Source: CAD feature listing. Evaluate the final solid. Frame: model axes, mm. A direction names the side the tool comes from. Give positions to 0.01 mm unless a question says otherwise; leave off trailing zeros. Loops run counter-clockwise (first coordinate to the right, second up) from the corner with the lowest first, then second, coordinate; pieces in that order, holes last. Notation, with made-up numbers: M 73.25,85.5 L 93.25,85.5 A16 cw 93.25,112.5 Z; hole C -6,22.5 d8. An arc over 180 degrees is marked long. Put each result on its own line as item: value.
from build123d import *

# Parameters (mm, degrees)
SKIZZE2_W                       = 113.5
SKIZZE2_H                       = 71
AUFSATZ_LINEAR_AUSTRAGEN1_DEPTH = 1.3
AUFSATZ_LINEAR_START            = -0.9
SKIZZE3_W                       = 120.5
SKIZZE3_H                       = 77.2
AUFSATZ_LINEAR_AUSTRAGEN2_DEPTH = 0.4
SKIZZE4_W                       = 107.4
SKIZZE4_H                       = 65
SCHNITT_LINEAR_AUSTRAGEN1_DEPTH = 103.975737434
VERRUNDUNG1_R                   = 1.5
VERRUNDUNG2_R                   = 3.3
VERRUNDUNG3_R                   = 3
SKIZZE5_R                       = 2.9
SCHNITT_LINEAR_AUSTRAGEN2_DEPTH = 103.975737434


with BuildPart() as part:
    # Skizze2 → Aufsatz-Linear austragen1 (new body)
    with BuildSketch(Plane.XY.offset(19.9)):
        with Locations((0, 46.4)):
            Rectangle(SKIZZE2_W, SKIZZE2_H)
    extrude(amount=-AUFSATZ_LINEAR_AUSTRAGEN1_DEPTH)

    # Skizze3 → Aufsatz-Linear austragen2 (add)
    with BuildSketch(Plane.XY.offset(19.9).offset(AUFSATZ_LINEAR_START)):
        with Locations((0, 44.9)):
            Rectangle(SKIZZE3_W, SKIZZE3_H)
    extrude(amount=-AUFSATZ_LINEAR_AUSTRAGEN2_DEPTH)

    # Skizze4 → Schnitt-Linear austragen1 (cut, through all)
    with BuildSketch(Plane.XY.offset(19.9)):
        with Locations((0, 46.4)):
            Rectangle(SKIZZE4_W, SKIZZE4_H)
    extrude(amount=-SCHNITT_LINEAR_AUSTRAGEN1_DEPTH, mode=Mode.SUBTRACT)

    # Verrundung1
    verrundung1_edges = [part.edges().sort_by_distance(p)[0] for p in [
        (56.75, 81.9, 19.45),
        (-56.75, 81.9, 19.45),
    ]]
    fillet(verrundung1_edges, radius=VERRUNDUNG1_R)

    # Verrundung2
    verrundung2_edges = [part.edges().sort_by_distance(p)[0] for p in [
        (-56.75, 10.9, 19.45),
        (56.75, 10.9, 19.45),
    ]]
    fillet(verrundung2_edges, radius=VERRUNDUNG2_R)

    # Verrundung3
    verrundung3_edges = [part.edges().sort_by_distance(p)[0] for p in [
        (60.25, 83.5, 18.8),
        (60.25, 6.3, 18.8),
        (-60.25, 6.3, 18.8),
        (-60.25, 83.5, 18.8),
    ]]
    fillet(verrundung3_edges, radius=VERRUNDUNG3_R)

    # Skizze5 → Schnitt-Linear austragen2 (cut, through all)
    with BuildSketch(Plane.XY.offset(19.9)):
        with Locations((20.5, 85.070858308)):
            Circle(SKIZZE5_R)
        with Locations((-20.5, 85.1)):
            Circle(SKIZZE5_R)
    extrude(amount=-SCHNITT_LINEAR_AUSTRAGEN2_DEPTH, mode=Mode.SUBTRACT)


solid = part.part
1. Material intervals for line 1 (X direction, y = 25, z = 19.35); line 2 (Y direction, x = -37, z = 18.85); line 3 (Y direction, x = 1, z = 19.7), sorted ascending. Write a range as from..to.
Found:
line 1: -56.75..-53.7, 53.7..56.75
line 2: 6.3..13.9, 78.9..83.5
line 3: 10.9..13.9, 78.9..81.9
2. Section query C-C (y = 45.5). Output: boundary loops of the cut face in (x, z), plus the area to 3 significant figures.
Found:
outline: M -60.25,18.6 L -53.7,18.6 L -53.7,19.9 L -56.75,19.9 L -56.75,19 L -60.25,19 Z; M 53.7,18.6 L 60.25,18.6 L 60.25,19 L 56.75,19 L 56.75,19.9 L 53.7,19.9 Z
area: 10.7 mm^2
3. Access query for faces 1 (the flat face through (0, 8, 19)), 2 (the cylindrical face through (59.35, 7.16, 18.8)), 3 (the cylindrical face through (-55.809, 11.892, 19.444)), 4 (the cylindrical face through (59.35, 82.64, 18.8)), 5 (the cylindrical face through (55.758, 11.841, 19.444)). Directions: +Z, -Z, +X, -X, +Y, -Y. A direction counts if a zero-diameter tool reaches every point of the face in a straight line with its end or side. Return the directions, or none.
Found:
face 1: +Z
face 2: +Z, -Z, +X, -Y
face 3: +Z, -X, -Y
face 4: +Z, -Z, +X, +Y
face 5: +Z, +X, -Y
4. Section query A-A (x = -28). Output: boundary loops of the cut face in (y, z), plus the area to 3 significant figures.
Found:
outline: M 6.3,18.6 L 13.9,18.6 L 13.9,19.9 L 10.9,19.9 L 10.9,19 L 6.3,19 Z; M 78.9,18.6 L 83.5,18.6 L 83.5,19 L 81.9,19 L 81.9,19.9 L 78.9,19.9 Z
area: 10.3 mm^2
5. Contact query for a flat-ended pin moving along its axis: P1, Ø0.7, axis at y = 54, z = 19.5, coming from the +X side. Output: stop coordinate, or through.
Found:
P1: x = 56.75
6. Section query B-B (z = 19.7). Output: boundary loops of the cut face in (x, y).
Found:
outline: M -56.75,14.2 A3.3 ccw -53.45,10.9 L 53.45,10.9 A3.3 ccw 56.75,14.2 L 56.75,80.4 A1.5 ccw 55.25,81.9 L -55.25,81.9 A1.5 ccw -56.75,80.4 Z; hole M -53.7,13.9 L 53.7,13.9 L 53.7,78.9 L -53.7,78.9 Z
